Could you check a few things on this model? Use its own coordinates, in mm. Face numbers are marked on the shaded views. A direction names the side the tool comes from. Round coordinates to 2 decimals unless told otherwise and drop trailing zeros. Write each loop counter-clockwise with the first axis right and the second up, starting at its lowest first coordinate (ties: lowest second). Pieces come first, ordered by that corner, then holes. Notation, with made-up numbers: (8.25, -19.75) -> (66.25, -19.75) arc R27 ccw to (66.25, 12.25) -> close; hole circle Ø4 at (0, 64). An arc over 180 degrees is marked (long way). Answer in a Markdown table with one row per item. Add a question column.
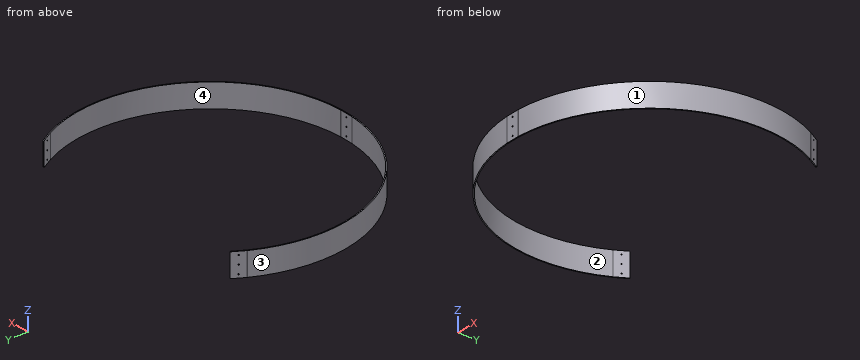
```python
from build123d import *

# Parameters (mm, degrees)
PAD001_DEPTH          = 70
SKETCH007_R           = 1.7
POCKET002_DEPTH       = 2438.582526
POLARPATTERN001_COUNT = 3
POCKET003_DEPTH       = 2494.311679


with BuildPart() as part:
    # Sketch006 → Pad001 (new body)
    with BuildSketch(Plane.XY):
        with BuildLine():
            ThreePointArc((20.253569, -398.856102), (345.928021, -199.575052), (355.430597, 182.113941))
            ThreePointArc((355.430597, 182.113941), (355.372093, 182.224683), (355.310833, 182.333925))
            Line((355.310833, 182.333925), (335.436031, 216.758093))
            Line((335.436031, 216.758093), (338.034107, 218.258093))
            Line((338.034107, 218.258093), (357.90891, 183.833925))
            ThreePointArc((358.100532, 183.48195), (358.006925, 183.659138), (357.90891, 183.833925))
            ThreePointArc((20.40571, -401.852241), (348.526574, -201.074226), (358.100532, 183.48195))
            ThreePointArc((20, -401.862536), (20.20292, -401.859962), (20.40571, -401.852241))
            Line((-20, -401.862536), (20, -401.862536))
            ThreePointArc((-20.40571, -401.852241), (-20.20292, -401.859962), (-20, -401.862536))
            ThreePointArc((-358.100532, 183.48195), (-348.526574, -201.074226), (-20.40571, -401.852241))
            ThreePointArc((-357.90891, 183.833925), (-358.006925, 183.659138), (-358.100532, 183.48195))
            Line((-357.90891, 183.833925), (-338.034107, 218.258093))
            Line((-338.034107, 218.258093), (-335.436031, 216.758093))
            Line((-355.310833, 182.333925), (-335.436031, 216.758093))
            ThreePointArc((-355.310833, 182.333925), (-355.372093, 182.224683), (-355.430597, 182.113941))
            ThreePointArc((-355.430597, 182.113941), (-345.928021, -199.575052), (-20.253569, -398.856102))
            ThreePointArc((-20.253569, -398.856102), (-20.126825, -398.860927), (-20, -398.862536))
            Line((-20, -398.862536), (20, -398.862536))
            ThreePointArc((20, -398.862536), (20.126825, -398.860927), (20.253569, -398.856102))
        make_face()
    extrude(amount=PAD001_DEPTH)

    # Sketch007 → Pocket002 (cut, through all)
    with BuildSketch(Plane.XZ):
        with Locations((0, 35)):
            Circle(SKETCH007_R)
        with Locations((0, 60)):
            Circle(SKETCH007_R)
        with Locations((0, 10)):
            Circle(SKETCH007_R)
    pocket002 = extrude(amount=POCKET002_DEPTH, mode=Mode.SUBTRACT)

    # PolarPattern001: Pocket002 ×3 about axis
    polarpattern001_axis = Axis((0, 0, 0), (0, 0, 1))
    for i in range(1, POLARPATTERN001_COUNT):
        add(pocket002.rotate(polarpattern001_axis, i * 360 / POLARPATTERN001_COUNT), mode=Mode.SUBTRACT)

    # Sketch008 → Pocket003 (cut, through all)
    with BuildSketch(Plane(origin=(0, 0, 0), x_dir=(0.5, -0.866025, 0), z_dir=(-0.866025, -0.5, 0))):
        with BuildLine():
            ThreePointArc((-20, 2.000018), (-19.414214, 0.585786), (-17.999982, 0))
            Line((-20, 0), (-17.999982, 0))
            Line((-20, 2.000018), (-20, 0))
        make_face()
        with BuildLine():
            ThreePointArc((-17.999982, 70), (-19.414209, 69.414209), (-20, 67.999982))
            Line((-20, 67.999982), (-20, 70))
            Line((-20, 70), (-17.999982, 70))
        make_face()
    pocket003 = extrude(amount=-POCKET003_DEPTH, mode=Mode.SUBTRACT)

    # Mirrored002: Pocket003 across YZ
    add(pocket003.mirror(Plane.YZ), mode=Mode.SUBTRACT)


solid = part.part
```
(1) If we mould it in two halves opening along Y, with no side actions, what happens to the marked faces 3 and 4? For each: pulls with the +Y half, pulls with the -Y half, needs draft (parallel to the pull), parting line crosses it, or undercut.
(2) Suppose I cut it at D-D, the plane x = 219. Please give me the cut outline in (y, z).
(3) Suppose I cut it at B-B, the plane z = 46.5. Please give me the cut outline in (x, y), then the cut area to 3 significant figures.
(4) Suppose I cut it at A-A, the plane y = -199.5. Please give me the cut outline in (x, z).
(5) I need wall thicknesses on L1, parallel to Z at x = 0, y = -400; L2, parallel to X at y = -369, z = 59.5; L3, parallel to X at y = 129.5, z = 24. Which ranges of each line are inside material? Lowest first, please.
(6) On a 3-axis mill with a long thin cutter (end or side, diameter ignored), from which of +Z, -Z, +X, -X, +Y, -Y can I reach the whole of each face in a straight line? I mean the marked faces 1 and 2. Say none if no direction works.
(7) For P1, Ø2, axis at y = 0.5, z = 54.5, coming from the +X side; P2, Ø4.5, axis at x = 0, z = 10, coming from the +Y side; P3, Ø2, axis at y = -294.5, z = 28.5, coming from the -X side, each with a flat end and sliding along its axis, tell me the tip position at first contact or that it passes through.
(8) Suppose I cut it at C-C, the plane y = -97.5. Please give me the cut outline in (x, z), then the cut area to 3 significant figures.
Response:
| question | item | result |
|---|---|---|
| 1 | face 3 | parting line crosses it |
| 1 | face 4 | undercut |
| 2 | outline | (-337.55, 0) -> (-333.97, 0) -> (-333.97, 70) -> (-337.55, 70) -> close |
| 3 | outline | (-358.1, 183.48) arc R402.37 ccw to (-20.41, -401.85) arc R8 ccw to (-20, -401.86) -> (20, -401.86) arc R8 ccw to (20.41, -401.85) arc R402.37 ccw to (358.1, 183.48) arc R8 ccw to (357.91, 183.83) -> (338.03, 218.26) -> (335.44, 216.76) -> (355.31, 182.33) arc R5 cw to (355.43, 182.11) arc R399.37 cw to (20.25, -398.86) arc R5 cw to (20, -398.86) -> (-20, -398.86) arc R5 cw to (-20.25, -398.86) arc R399.37 cw to (-355.43, 182.11) arc R5 cw to (-355.31, 182.33) -> (-335.44, 216.76) -> (-338.03, 218.26) -> (-357.91, 183.83) arc R8 ccw to start |
| 3 | area | 5,160 mm² |
| 4 | outline | (-349.43, 0) -> (-345.97, 0) -> (-345.97, 70) -> (-349.43, 70) -> close; (345.97, 0) -> (349.43, 0) -> (349.43, 70) -> (345.97, 70) -> close |
| 5 | L1 | 0 to 8.3, 11.7 to 33.3, 36.7 to 58.3, 61.7 to 70 |
| 5 | L2 | -160.44 to -152.76, 152.76 to 160.44 |
| 5 | L3 | -380.96 to -377.79, 377.79 to 380.96 |
| 6 | face 1 | +Z, -Z, +X |
| 6 | face 2 | +Z, -Z |
| 7 | P1 | x = 402.37 |
| 7 | P2 | y = -398.86 |
| 7 | P3 | x = -275.24 |
| 8 | outline | (-390.38, 0) -> (-387.29, 0) -> (-387.29, 70) -> (-390.38, 70) -> close; (387.29, 0) -> (390.38, 0) -> (390.38, 70) -> (387.29, 70) -> close |
| 8 | area | 433 mm² |
